Here's the drawing with two shaded views (mm, measured from the low corner). I have some questions. A direction names the side the tool comes from. Give positions to 0.01 mm unless a question says otherwise; leave off trailing zeros. Loops run counter-clockwise (first coordinate to the right, second up) from the corner with the lowest first, then second, coordinate; pieces in that order, holes last.
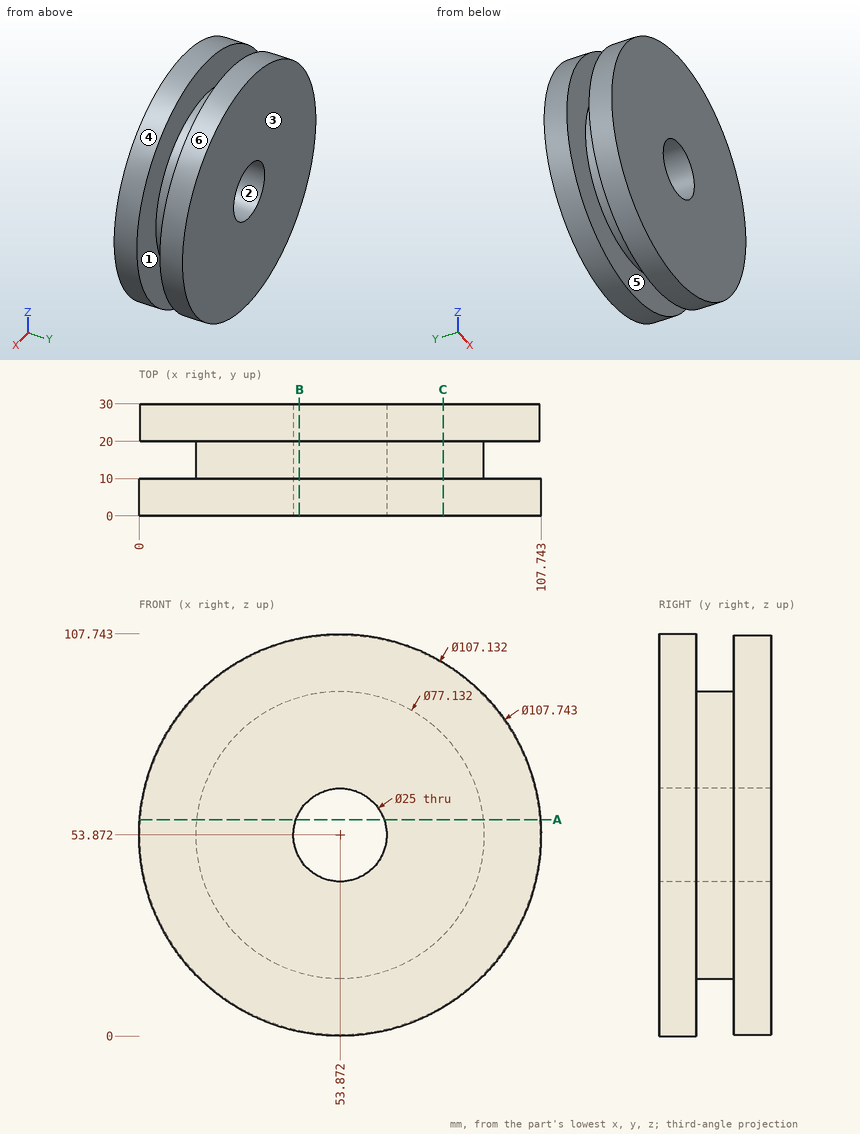
(1) Suppose I cut it at B-B on x = 43. List the corners of the cut face in (y, z) for me (1 decimal).
Returned:
outline: (0, 1.1) - (10, 1.1) - (10, 16.9) - (20, 16.9) - (20, 1.4) - (30, 1.4) - (30, 47.7) - (0, 47.7) - close; (0, 60) - (30, 60) - (30, 106.3) - (20, 106.3) - (20, 90.9) - (10, 90.9) - (10, 106.6) - (0, 106.6) - close
(2) Thinking about a two-plate mould opening in Y: for the marked faces 1, 2 and 3, which applies, pulls with the +Y half, pulls with the -Y half, needs draft (parallel to the pull), parting line crosses it, or undercut?
Returned:
face 1: undercut
face 2: needs draft
face 3: pulls with the +Y half
(3) Please list where these lines run through material, in increasing order: probe 1 along Y at (x, z) = (31, 14.5); probe 2 along X at (y, z) = (14.25, 45) (1 decimal); probe 3 along Z at (x, y) = (45.5, 11.5) (1 decimal).
Returned:
probe 1: y = 0 to 10, 20 to 30
probe 2: x = 16.3 to 45.1, 62.7 to 91.4
probe 3: z = 16.2 to 44.6, 63.2 to 91.5
(4) Suppose I cut it at A-A on z = 58. List the corners of the cut face in (x, y) for me (1 decimal).
Returned:
outline: (0.2, 0) - (42.1, 0) - (42.1, 30) - (0.5, 30) - (0.5, 20) - (15.5, 20) - (15.5, 10) - (0.2, 10) - close; (65.7, 0) - (107.6, 0) - (107.6, 10) - (92.2, 10) - (92.2, 20) - (107.3, 20) - (107.3, 30) - (65.7, 30) - close
(5) Suppose I cut it at C-C on x = 81.5. List the corners of the cut face in (y, z) for me (1 decimal).
Returned:
outline: (0, 7.6) - (10, 7.6) - (10, 27) - (20, 27) - (20, 8) - (30, 8) - (30, 99.8) - (20, 99.8) - (20, 80.8) - (10, 80.8) - (10, 100.1) - (0, 100.1) - close
(6) Which directions (+Z, -Z, +X, -X, +Y, -Y) give clear straight access to the entire face, cutting with the end or side of a thin tool? Please do the marked faces 4, 5 and 6.
Returned:
face 4: +Y, -Y
face 5: none
face 6: +Y
(7) Will these pins go through, and if not, where does the flat tip stop? P1, Ø5, axis at y = 13, z = 60, coming from the -X side; P2, Ø8, axis at x = 44, y = 16.5, coming from the +Z side; P3, Ø2, axis at y = 10, z = 30, coming from the +X side.
Returned:
P1: stops at x = 15.48
P2: stops at z = 106.85
P3: stops at x = 102.65
